from build123d import *

# Parameters (mm, degrees)
SKETCH1_W           = 330
SKETCH1_H           = 95
BOSS_EXTRUDE1_DEPTH = 85
SKETCH3_R           = 11
CUT_EXTRUDE2_DEPTH  = 150


with BuildPart() as part:
    # Sketch1 → Boss-Extrude1 (new body)
    with BuildSketch(Plane.YZ):
        with Locations((0, -36)):
            Rectangle(SKETCH1_W, SKETCH1_H)
    extrude(amount=BOSS_EXTRUDE1_DEPTH)

    # Sketch3 → Cut-Extrude2 (cut)
    with BuildSketch(Plane.XY.offset(11.5)):
        with Locations((42.5, 125)):
            Circle(SKETCH3_R)
        with Locations(Location((42.5, -125, 0), (0, 0, 270))):
            Circle(SKETCH3_R)
    extrude(amount=-CUT_EXTRUDE2_DEPTH, mode=Mode.SUBTRACT)


solid = part.part
Verification items for the finished model (mm, model axes). Give positions to 0.01 mm unless a question says otherwise; leave off trailing zeros. Write each loop counter-clockwise with the first axis right and the second up, starting at its lowest first coordinate (ties: lowest second). Pieces come first, ordered by that corner, then holes.
(1) Gauge pin test, flat end, axial feed: pin 1 (1 mm diameter, centred on y = -18, z = -55, fed in from -X). Record the tip position at first contact, or that the pin passes through.
(2) Material ranges on line 1 (Y direction, x = 42, z = -40); line 2 (X direction, y = -125, z = -34); line 3 (Y direction, x = 51, z = -29), recorded low to high.
(3) Cross-section at C-C (z = -40.5). Enter the section's corners in (x, y).
(4) Mould release check, pull along X, two halves, no side actions. Record for faces 1 (the face through (0, -2, -35)), 2 (the face through (42, -2, -83.5)), 3 (the face through (85, -2, -35)), 4 (the face through (41.068, 135.906, -35.335)): +X half, -X half, draft (parallel to the pull), parting line (faces both ways), or undercut.
(5) Cross-section at B-B (x = 42.5). Enter the section's corners in (y, z), plus the area to 3 significant figures.
(6) Cross-section at A-A (y = 125). Enter the section's corners in (x, z).
(7) Cross-section at D-D (y = -124.5). Enter the section's corners in (x, z).
Worked out:
1. pin 1: stops at x = 0
2. line 1: y = -165 to -135.99, -114.01 to 114.01, 135.99 to 165
2. line 2: x = 0 to 31.5, 53.5 to 85
2. line 3: y = -165 to -131.98, -118.02 to 118.02, 131.98 to 165
3. outline: (0, -165) - (85, -165) - (85, 165) - (0, 165) - close; hole circle Ø22 at (42.5, -125); hole circle Ø22 at (42.5, 125)
4. face 1: -X half
4. face 2: draft
4. face 3: +X half
4. face 4: undercut
5. outline: (-165, -83.5) - (-136, -83.5) - (-136, 11.5) - (-165, 11.5) - close; (-114, -83.5) - (114, -83.5) - (114, 11.5) - (-114, 11.5) - close; (136, -83.5) - (165, -83.5) - (165, 11.5) - (136, 11.5) - close
5. area: 27,200 mm2
6. outline: (0, -83.5) - (31.5, -83.5) - (31.5, 11.5) - (0, 11.5) - close; (53.5, -83.5) - (85, -83.5) - (85, 11.5) - (53.5, 11.5) - close
7. outline: (0, -83.5) - (31.51, -83.5) - (31.51, 11.5) - (0, 11.5) - close; (53.49, -83.5) - (85, -83.5) - (85, 11.5) - (53.49, 11.5) - close
